from build123d import *

# Parameters (mm, degrees)
CYLINDER814_R               = 1.5
CYLINDER814_DEPTH           = 20
CYLINDER814_PLACEMENT_ANGLE = 135
CYLINDER815_R               = 1.5
CYLINDER815_DEPTH           = 20
CYLINDER815_PLACEMENT_ANGLE = 45
CYLINDER812_R               = 3
CYLINDER812_DEPTH           = 3
CYLINDER812_PLACEMENT_ANGLE = 135
CYLINDER813_R               = 3
CYLINDER813_DEPTH           = 3
CYLINDER813_PLACEMENT_ANGLE = 45
BOX316_W                    = 30.2
BOX316_H                    = 30.2
BOX316_DEPTH                = 100
BOX316_PLACEMENT_ANGLE      = 45
CYLINDER806_R               = 27
CYLINDER806_DEPTH           = 3
CHAMFER001_SIZE             = 1


with BuildPart() as obj1:
    # Cylinder814 → Cylinder814 (new body)
    with BuildSketch(Plane.XY):
        Circle(CYLINDER814_R)
    extrude(amount=CYLINDER814_DEPTH)


with BuildPart() as obj1_1:
    # Cylinder814 placement: moved
    add(obj1.part.moved(Location((-14.142136, 14.142136, -30))).rotate(Axis((-14.142136, 14.142136, -30), (0, 0, 1)), CYLINDER814_PLACEMENT_ANGLE))


with BuildPart() as compound724:
    # Cylinder815 → Cylinder815 (new body)
    with BuildSketch(Plane.XY):
        Circle(CYLINDER815_R)
    extrude(amount=CYLINDER815_DEPTH)


with BuildPart() as compound724_1:
    # Cylinder815 placement: moved
    add(compound724.part.moved(Location((14.142136, -14.142136, -30))).rotate(Axis((14.142136, -14.142136, -30), (0, 0, -1)), CYLINDER815_PLACEMENT_ANGLE))

    # Compound724: union obj1
    add(obj1_1.part)


with BuildPart() as obj2:
    # Cylinder812 → Cylinder812 (new body)
    with BuildSketch(Plane.XY):
        Circle(CYLINDER812_R)
    extrude(amount=CYLINDER812_DEPTH)


with BuildPart() as obj2_1:
    # Cylinder812 placement: moved
    add(obj2.part.moved(Location((-14.142136, 14.142136, -30))).rotate(Axis((-14.142136, 14.142136, -30), (0, 0, 1)), CYLINDER812_PLACEMENT_ANGLE))


with BuildPart() as compound723:
    # Cylinder813 → Cylinder813 (new body)
    with BuildSketch(Plane.XY):
        Circle(CYLINDER813_R)
    extrude(amount=CYLINDER813_DEPTH)


with BuildPart() as compound723_1:
    # Cylinder813 placement: moved
    add(compound723.part.moved(Location((14.142136, -14.142136, -30))).rotate(Axis((14.142136, -14.142136, -30), (0, 0, -1)), CYLINDER813_PLACEMENT_ANGLE))

    # Compound723: union obj2
    add(obj2_1.part)


with BuildPart() as compound723_2:
    # Compound723 placement: moved
    add(compound723_1.part.moved(Location((0, 0, 17))))


with BuildPart() as krychle316:
    # Box316 → Box316 (new body)
    with BuildSketch(Plane.XY):
        with Locations((15.1, 15.1)):
            Rectangle(BOX316_W, BOX316_H)
    extrude(amount=BOX316_DEPTH)


with BuildPart() as krychle316_1:
    # Box316 placement: moved
    add(krychle316.part.moved(Location((0, -21.354625, -30))).rotate(Axis((0, -21.354625, -30), (0, 0, 1)), BOX316_PLACEMENT_ANGLE))


with BuildPart() as g_midi_belt_wheel_front:
    # Cylinder806 → Cylinder806 (new body)
    with BuildSketch(Plane.XY.offset(-15)):
        Circle(CYLINDER806_R)
    extrude(amount=CYLINDER806_DEPTH)

    # Cut341: cut Krychle316
    add(krychle316_1.part, mode=Mode.SUBTRACT)

    # Chamfer001
    chamfer001_edges = [g_midi_belt_wheel_front.edges().sort_by_distance(p)[0] for p in [
        (-27, 0, -15),
    ]]
    chamfer(chamfer001_edges, length=CHAMFER001_SIZE)

    # Cut345: cut Compound723
    add(compound723_2.part, mode=Mode.SUBTRACT)

    # Cut346: cut Compound724
    add(compound724_1.part, mode=Mode.SUBTRACT)


with BuildPart() as g_midi_belt_wheel_front_1:
    # Cut346 placement: moved
    add(g_midi_belt_wheel_front.part.moved(Location((0, 0, 54))))


solid = g_midi_belt_wheel_front_1.part
Check sheet for the modelled part. Datum: model origin and axes. Units: mm. A direction names the side the tool comes from. Give positions to 0.01 mm unless a question says otherwise; leave off trailing zeros. Loops run counter-clockwise (first coordinate to the right, second up) from the corner with the lowest first, then second, coordinate; pieces in that order, holes last. Notation, with made-up numbers: M 35,-5.75 L 64,-5.75 A29 cw 64,15.25 Z; hole C 49,18 d4. An arc over 180 degrees is marked long. Answer as a JSON object with one key per item and string values. Group by question number.
Q1. Cross-section at A-A on z = 40.5. Record the cut outline in (x, y), then the cut area to 3 significant figures.
Q2. Go/stop test with flat-tipped pins: P1, Ø1.8, axis at x = 14.5, y = -13.5, coming from the +Z side; P2, Ø1.5, axis at y = 7, z = 40.5, coming from the -X side. Record where each tip stops, or that it passes through.
Q3. Material ranges on line 1 along X through (y, z) = (-22, 40.3); line 2 along X through (y, z) = (-4, 40.3); line 3 along X through (y, z) = (15.5, 39.9), recorded low to high. Write a range as [from, to].
Q4. Release check for a two-part mould opening along Y. For faces 1 (the flat face through (11.6, -11.6, 42)), 2 (the cylindrical face through (-5.85, -26.36, 40.99)), 3 (the flat face through (-10.528, -10.827, 40.479)) record: released by +Y, released by -Y, zero draft, split by the parting line, or undercut.
Q5. Access from +Z, -Z, +X, -X, +Y, -Y to the whole of each face (thin tool, end or side, straight path). Record for faces 4 (the flat face through (10.827, 10.528, 40.479)), 5 (the flat face through (11, -11, 39)), 6 (the cylindrical face through (-11.61, 15.75, 41.49)).
Evaluation:
{
 "1": {"outline": "C 0,0 d54; hole M -21.35,0 L 0,-21.35 L 21.35,0 L 0,21.35 Z; hole C -14.14,14.14 d3; hole C 14.14,-14.14 d3", "area": "1,360 mm2"},
 "2": {"P1": "stops at z = 41", "P2": "stops at x = -26.27"},
 "3": {"line 1": "x = [-15.65, 15.65]", "line 2": "x = [-26.7, -17.35], [17.35, 26.7]", "line 3": "x = [-21.99, -14.78], [-13.5, -5.85], [5.85, 21.99]"},
 "4": {"face 1": "zero draft", "face 2": "split by the parting line", "face 3": "undercut"},
 "5": {"face 4": "+Z, -Z", "face 5": "-Z, +X, -X, +Y, -Y", "face 6": "+Z"}
}
